Here's how the part is built. I have some questions about the finished solid (model axes, mm). Face numbers are marked on the shaded views. A direction names the side the tool comes from. Coordinates: 2 decimals unless noted, no trailing zeros. Write each loop counter-clockwise with the first axis right and the second up, starting at its lowest first coordinate (ties: lowest second). Pieces come first, ordered by that corner, then holes. Notation, with made-up numbers: (6, 78) -> (22, 78) arc R19 ccw to (22, 111) -> close; hole circle Ø7 at (-32, 55.25). An arc over 180 degrees is marked (long way). Use a Markdown table: item, result. Add a question column.
Item 1: Imagine slicing it at A-A, the plane z = 0. Write out the boundary of the cut face in (x, y), and give its area (3 significant figures).
Item 2: Imagine slicing it at B-B, the plane x = 0. Write out the boundary of the cut face in (y, z).
Item 3: If we mould it in two halves opening along Y, with no side actions, what happens to the marked faces 3, 4 and 5? For each: pulls with the +Y half, pulls with the -Y half, needs draft (parallel to the pull), parting line crosses it, or undercut.
Item 4: Will these pins go through, and if not, where does the flat tip stop? pin 1 Ø6 at (x, z) = (-32.5, -5) entering from -Y; pin 2 Ø3 at (y, z) = (119, -49.5) entering from +X; pin 3 Ø2 at (x, y) = (46, 48.5) entering from +Z; pin 4 Ø5.5 at (y, z) = (34, -27.5) entering from +X.
Item 5: Imagine slicing it at C-C, the plane y = 247.5. Write out the boundary of the cut face in (x, z), and give its area (3 significant figures).
Item 6: If I drill on line 1 along X through (y, z) = (100, 0); line 2 along Z through (x, y) = (-25, 171), over which ranges is the centre line in solid material (lowest first)? Write a range as from..to.
Item 7: Imagine slicing it at D-D, the plane z = 16.5. Count the separate pieces of the cut face and the enclosed holes in it, and give its area (3 significant figures).
Item 8: On a 3-axis mill with a long thin cutter (end or side, diameter ignored), from which of +Z, -Z, +X, -X, +Y, -Y can I reach the whole of each face in a straight line? I mean the marked faces 1 and 2. Say none if no direction works.
```python
from build123d import *

# Parameters (mm, degrees)
SKETCH3_R               = 68
BOSS_EXTRUDE1_DEPTH     = 300
SHELL1_T                = -5
CUT_EXTRUDE1_DEPTH      = 316.036505821
CUT_EXTRUDE1_DEPTH_BACK = 316.036505821
CUT_EXTRUDE2_START      = -116
CUT_EXTRUDE2_DEPTH      = 116


with BuildPart() as part:
    # Sketch3 → Boss-Extrude1 (new body)
    with BuildSketch(Plane(origin=(0, 0, 0), x_dir=(1, 0, 0), z_dir=(0, 1, 0))):
        with Locations(Location((0, 0, 0), (0, 0, 270))):
            Circle(SKETCH3_R)
    extrude(amount=BOSS_EXTRUDE1_DEPTH)

    # Sketch5 → Cut-Revolve1 (revolve, cut)
    with BuildSketch(Plane.XY, mode=Mode.PRIVATE) as cut_revolve1_sk:
        Polygon((-58, 0), (-68, 0), (-68, 40), align=None)
    revolve(cut_revolve1_sk.sketch.rotate(Axis((0, 300, 0), (0, -1, 0)), 270), axis=Axis((0, 300, 0), (0, -1, 0)), mode=Mode.SUBTRACT)

    # Shell1
    shell1_openings = [part.faces().sort_by_distance(p)[0] for p in [
        (0, 0, 0),
    ]]
    offset(amount=SHELL1_T, openings=shell1_openings, kind=Kind.INTERSECTION)

    # Sketch6 → Cut-Extrude1 (cut, two sides: drawn at the far end of the back side and taken through both)
    with BuildSketch(Plane.XY.offset(-CUT_EXTRUDE1_DEPTH_BACK)):
        Polygon((-68, 70), (-68, 30), (-58, 20), (-58, 60), align=None)
        Polygon((68, 30), (58, 20), (58, 60), (68, 70), align=None)
    extrude(amount=CUT_EXTRUDE1_DEPTH + CUT_EXTRUDE1_DEPTH_BACK, mode=Mode.SUBTRACT)

    # Sketch7 → Cut-Extrude2 (cut)
    with BuildSketch(Plane.ZY.offset(58).offset(CUT_EXTRUDE2_START)):
        Polygon((-35.496478699, 60), (35.496478699, 60), (35.496478699, 40), (24.596747752, 20), (-24.596747752, 20), (-35.496478699, 40), align=None)
    extrude(amount=CUT_EXTRUDE2_DEPTH, mode=Mode.SUBTRACT)


solid = part.part
```
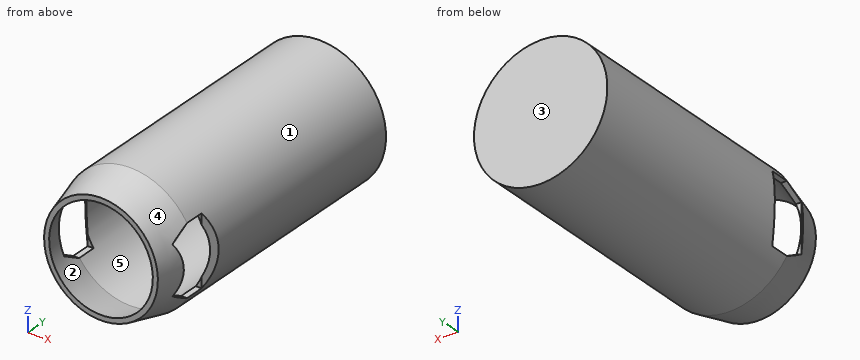
Ans:
| question | item | result |
|---|---|---|
| 1 | outline | (-68, 70) -> (-63, 65) -> (-63, 295) -> (63, 295) -> (63, 65) -> (68, 70) -> (68, 300) -> (-68, 300) -> close; (-64.67, 26.67) -> (-58, 0) -> (-52.85, 0) -> (-57.85, 20) -> (-58, 20) -> close; (52.85, 0) -> (58, 0) -> (64.67, 26.67) -> (58, 20) -> (57.85, 20) -> close |
| 1 | area | 3,190 mm^2 |
| 2 | outline | (0, -58) -> (40, -68) -> (300, -68) -> (300, 68) -> (40, 68) -> (0, 58) -> (0, 52.85) -> (40.62, 63) -> (295, 63) -> (295, -63) -> (40.62, -63) -> (0, -52.85) -> close |
| 3 | face 3 | pulls with the +Y half |
| 3 | face 4 | pulls with the -Y half |
| 3 | face 5 | undercut |
| 4 | pin 1 | stops at y = 295 |
| 4 | pin 2 | stops at x = 48.17 |
| 4 | pin 3 | stops at z = 50.98 |
| 4 | pin 4 | passes through |
| 5 | outline | circle Ø136 at (0, 0); hole circle Ø126 at (0, 0) |
| 5 | area | 2,060 mm^2 |
| 6 | line 1 | x = -68..-63, 63..68 |
| 6 | line 2 | z = -63.24..-57.83, 57.83..63.24 |
| 7 | separate pieces | 3 |
| 7 | enclosed holes | 0 |
| 7 | area | 3,260 mm^2 |
| 8 | face 1 | +Y, -Y |
| 8 | face 2 | none |
